Here's the drawing with two shaded views (mm, measured from the low corner). I have some questions. A direction names the side the tool comes from. Coordinates: 2 decimals unless noted, no trailing zeros. Write each loop counter-clockwise with the first axis right and the second up, starting at its lowest first coordinate (ties: lowest second). Pieces come first, ordered by that corner, then holes.
Item 1: For the marked faces 1, 2, 3 and 4, which set-ups out of +Z, -Z, +X, -X, +Y, -Y let a thin tool reach every point of the face, with its end or its side?
Item 2: If we section it at B-B (y = 5): Please give me the cut outline in (x, z).
Item 3: If I drill on line 1 (Y direction, x = 19.95, z = 78); line 2 (Z direction, x = 20, y = 108); line 3 (Z direction, x = 15.75, y = 93.5), over which ranges is the centre line in solid material (lowest first)?
Item 4: I'm going to push flat-ended pins straight in: pin 1 Ø0.6 at (x, z) = (11, 27) entering from +Y; pin 2 Ø3.5 at (x, z) = (7, 20) entering from +Y; pin 3 Ø1 at (x, z) = (13, 15) entering from -Y; pin 4 Ø6 at (x, z) = (13, 68.5) entering from +Y. Where does each tip first touch, or does it pass through?
Item 5: If we section it at D-D (z = 5): Please give me the cut outline in (x, y).
Item 6: If we section it at C-C (y = 108): Please give me the cut outline in (x, z).
Item 7: If we section it at A-A (z = 78): Please give me the cut outline in (x, y).
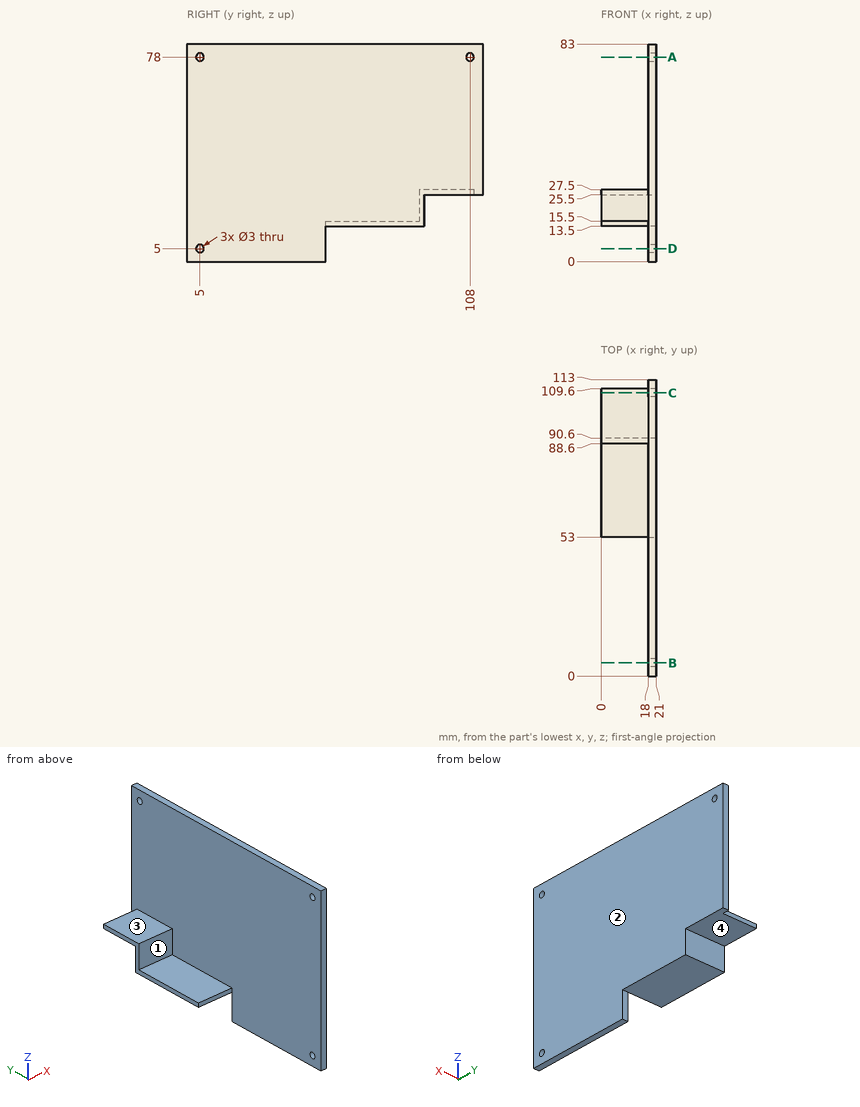
Answer list:
1. face 1: +Z, -X, -Y
1. face 2: +Z, -Z, +X, +Y, -Y
1. face 3: +Z, -X, +Y, -Y
1. face 4: -Z, +X, -X, +Y
2. outline: (18, 0) - (21, 0) - (21, 3.5) - (18, 3.5) - close; (18, 6.5) - (21, 6.5) - (21, 76.5) - (18, 76.5) - close; (18, 79.5) - (21, 79.5) - (21, 83) - (18, 83) - close
3. line 1: y = 0 to 3.5, 6.5 to 106.5, 109.5 to 113
3. line 2: z = 25.5 to 76.5, 79.5 to 83
3. line 3: z = 25.5 to 27.5
4. pin 1: stops at y = 109.6
4. pin 2: stops at y = 90.6
4. pin 3: stops at y = 53
4. pin 4: passes through
5. outline: (18, 0) - (21, 0) - (21, 3.5) - (18, 3.5) - close; (18, 6.5) - (21, 6.5) - (21, 53) - (18, 53) - close
6. outline: (0, 25.5) - (21, 25.5) - (21, 76.5) - (18, 76.5) - (18, 27.5) - (0, 27.5) - close; (18, 79.5) - (21, 79.5) - (21, 83) - (18, 83) - close
7. outline: (18, 0) - (21, 0) - (21, 3.5) - (18, 3.5) - close; (18, 6.5) - (21, 6.5) - (21, 106.5) - (18, 106.5) - close; (18, 109.5) - (21, 109.5) - (21, 113) - (18, 113) - close
